Here's how the part is built. I have some questions about the finished solid (model axes, mm). A direction names the side the tool comes from. Round coordinates to 2 decimals unless told otherwise and drop trailing zeros. Order: outer loops, then holes, each group sorted by start corner. A loop starts at its lowest first (then second) coordinate and runs counter-clockwise, first axis right, second up. Notation, with made-up numbers: M 0.25,9 L 54.25,9 A17 cw 54.25,27 Z; hole C -12.75,56.25 d10. An arc over 180 degrees is marked long. Use one line per item in the form item = value. Start each with the question number.
```python
from build123d import *

# Parameters (mm, degrees)
SKIZZE4_R            = 72.5
SKIZZE4_R_2          = 72
BASE_RING_DEPTH      = 17.9
ULTRASONIC_CUT_DEPTH = 105.081266326
ROTATION_I_COUNT     = 8
SCREW_BASE_DEPTH     = 5
SKIZZE7_R            = 1.5
SCREW_CENTER_DEPTH   = 104.338811836
SKIZZE7_3_R          = 1.5
HEX_NUT_DEPTH        = 2.5
KREISMUSTER2_COUNT   = 2


with BuildPart() as part:
    # Skizze4 → Base Ring (new body)
    with BuildSketch(Plane.XY):
        with Locations(Location((0, 0, 0), (0, 0, 180))):
            Circle(SKIZZE4_R)
        with Locations(Location((0, 0, 0), (0, 0, 180))):
            Circle(SKIZZE4_R_2, mode=Mode.SUBTRACT)
    extrude(amount=BASE_RING_DEPTH)

    # Skizze5 → Ultrasonic Cut (cut, through all)
    with BuildSketch(Plane(origin=(0, 0, 0), x_dir=(0, 0, -1), z_dir=(1, 0, 0))):
        with BuildLine():
            Line((-17.9, 4.5), (-48.848327202, 4.5))
            Line((-48.848327202, 4.5), (-48.848327202, 21.5))
            Line((-48.848327202, 21.5), (-17.9, 21.5))
            ThreePointArc((-17.9, 21.5), (-9.4, 13), (-17.9, 4.5))
        make_face()
        with BuildLine():
            Line((-17.9, -21.5), (-48.848327202, -21.5))
            Line((-48.848327202, -21.5), (-48.848327202, -4.5))
            Line((-48.848327202, -4.5), (-17.9, -4.5))
            ThreePointArc((-17.9, -4.5), (-9.4, -13), (-17.9, -21.5))
        make_face()
    ultrasonic_cut = extrude(amount=ULTRASONIC_CUT_DEPTH, mode=Mode.SUBTRACT)

    # Rotation I: Ultrasonic Cut ×8 about axis
    rotation_i_axis = Axis((0, 0, 17.9), (0, 0, -1))
    for i in range(1, ROTATION_I_COUNT):
        add(ultrasonic_cut.rotate(rotation_i_axis, i * 360 / ROTATION_I_COUNT), mode=Mode.SUBTRACT)

    # Skizze6 → Screw Base (add)
    with BuildSketch(Plane.XY):
        with BuildLine():
            Line((22.597553321, 63.701260458), (29.064710048, 61.022476431))
            ThreePointArc((29.064710048, 61.022476431), (24.491739671, 59.128290081), (22.597553321, 63.701260458))
        make_face()
        with BuildLine():
            ThreePointArc((24.287054845, 67.78007795), (27.55320713, 66.519326341), (30.754211572, 65.101293924))
            Line((30.754211572, 65.101293924), (29.064710048, 61.022476431))
            Line((29.064710048, 61.022476431), (22.597553321, 63.701260458))
            Line((22.597553321, 63.701260458), (24.287054845, 67.78007795))
        make_face()
    screw_base = extrude(amount=SCREW_BASE_DEPTH)

    # Skizze7 → Screw Center (cut, through all)
    with BuildSketch(Plane.XY.offset(5)):
        with Locations((25.831131685, 62.361868445)):
            Circle(SKIZZE7_R)
    screw_center = extrude(amount=-SCREW_CENTER_DEPTH, mode=Mode.SUBTRACT)

    # Skizze7<3> → Hex Nut (cut)
    with BuildSketch(Plane.XY.offset(5)):
        Polygon((29.122494691, 62.795184605), (27.101550385, 65.428930501), (23.810187379, 64.995614341), (22.539768678, 61.928552284), (24.560712984, 59.294806388), (27.85207599, 59.728122548), align=None)
        with Locations((25.831131685, 62.361868445)):
            Circle(SKIZZE7_3_R, mode=Mode.SUBTRACT)
    hex_nut = extrude(amount=-HEX_NUT_DEPTH, mode=Mode.SUBTRACT)

    # Kreismuster2: Screw Base, Screw Center, Hex Nut ×2 about axis
    kreismuster2_axis = Axis((0, 0, 0), (0, 0, 1))
    add([screw_base.rotate(kreismuster2_axis, i * 360 / KREISMUSTER2_COUNT) for i in range(1, KREISMUSTER2_COUNT)])
    add([screw_center.rotate(kreismuster2_axis, i * 360 / KREISMUSTER2_COUNT) for i in range(1, KREISMUSTER2_COUNT)], mode=Mode.SUBTRACT)
    add([hex_nut.rotate(kreismuster2_axis, i * 360 / KREISMUSTER2_COUNT) for i in range(1, KREISMUSTER2_COUNT)], mode=Mode.SUBTRACT)


solid = part.part
```
1) On a 3-axis mill with a long thin cutter (end or side, diameter ignored), from which of +Z, -Z, +X, -X, +Y, -Y can I reach the whole of each face in a straight line? I mean faces 4 (the flat face through (-29.92, -63.09, 2.46)), 5 (the flat face through (-66.7, -27.7, 17.9)), 6 (the flat face through (27.5, 65.3, 5)). Say none if no direction works.
2) If we section it at A-A on x = 0: Write out the boundary of the cut face in (y, z).
3) If we mould it in two halves opening along X, with no side actions, what happens to faces 1 (the cylindrical face through (13.1, -71.1, 9.4)), 2 (the flat face through (-51.2, -51, 17.9)), 3 (the cylindrical face through (-59.5, 41, 9.4))? For each: +X half, -X half, draft (parallel to the pull), parting line (faces both ways), or undercut.
4) If we section it at C-C on z = 11.5: Give the number of separate pieces and of enclosed holes in the cut face, then the cut area to 3 significant figures.
5) Will these pins go through, and if not, where does the flat tip stop? pin 1 Ø3 at (x, y) = (-26, -63) entering from +Z; pin 2 Ø3 at (y, z) = (-54, 10.5) entering from -X; pin 3 Ø2.5 at (x, y) = (26.5, 64.5) entering from +Z; pin 4 Ø1.5 at (x, y) = (52.5, -50) entering from -Z.
6) If I drill on line 1 (X direction, y = 63.5, z = 3.25); line 2 (Y direction, x = -53.5, z = 6), over which ranges is the centre line in solid material (lowest first)?
Completed:
q1.face_4 = +Z, -Z
q1.face_5 = +Z, +X, -X, +Y, -Y
q1.face_6 = +Z
q2.outline = M -72.5,0 L -72,0 L -72,17.9 L -72.5,17.9 Z; M 72,0 L 72.5,0 L 72.5,17.9 L 72,17.9 Z
q3.face_1 = undercut
q3.face_2 = draft
q3.face_3 = undercut
q4.separate_pieces = 16
q4.enclosed_holes = 0
q4.area = 136 mm²
q5.pin_1 = 2.5
q5.pin_2 = -50
q5.pin_3 = 5
q5.pin_4 = 0
q6.line_1 = -34.99 to -33.94, 22.52 to 23.19, 28.58 to 30.09, 33.94 to 34.99
q6.line_2 = -48.93 to -48.18, 48.18 to 48.93
